Read the model definition and answer for the solid it produces. Units are mm, in the model's axes. Give positions to 0.01 mm unless a question says otherwise; leave off trailing zeros. Loops run counter-clockwise (first coordinate to the right, second up) from the corner with the lowest first, then second, coordinate; pieces in that order, holes last.
(1) Find section A-A, the plane z = 0. Write down the section's boundary in (x, y).
(2) Find section C-C, the plane z = 9.75. Write down the section's boundary in (x, y).
(3) Determine the mould class of faces 1 (the face through (2.88, -7.936, 0.018)), 2 (the face through (5.842, -3, 3)) for opening direction Z: pulls with the +Z half, pulls with the -Z half, needs draft (parallel to the pull), parting line crosses it, or undercut.
(4) Find section D-D, the plane z = -5.25. Write down the section's boundary in (x, y).
(5) Straight lines are drawn through the part: probe 1 along Y at (x, z) = (1.75, 0); probe 2 along Y at (x, z) = (5.2, 9.25); probe 3 along Z at (x, y) = (5.15, -6.25). For each, find the intervals that lie inside material, in ascending order.
(6) Find section B-B, the plane y = -10.5. Write down the section's boundary in (x, z), then the cut area to 3 significant figures.
```python
from build123d import *

# Parameters (mm, degrees)
BASPROSKE_W         = 5.842
BASPROSKE_H         = 12.7
TOOTHCUT_DEPTH      = 19.886740428
TEETHCUTS_COUNT     = 10
TEETHCUTS_ANGLE     = 324
BORSKE_R            = 3.175
BORE_DEPTH          = 50.8000508
SKETCH1_R           = 3.175
SKETCH1_R_2         = 2.921
BOSS_EXTRUDE1_DEPTH = 5.842


with BuildPart() as part:
    # BasProSke → Base-Revolve (revolve)
    with BuildSketch(Plane(origin=(0, 0, 0), x_dir=(1, 0, 0), z_dir=(0, 1, 0)), mode=Mode.PRIVATE) as base_revolve_sk:
        with Locations((2.921, 6.35)):
            Rectangle(BASPROSKE_W, BASPROSKE_H)
    revolve(base_revolve_sk.sketch.rotate(Axis((-10, 0, 0), (1, 0, 0)), 180), axis=Axis((-10, 0, 0), (1, 0, 0)))

    # TooCutSke → ToothCut (cut, through all)
    with BuildSketch(Plane(origin=(0, 0, 0), x_dir=(0, 0, -1), z_dir=(1, 0, 0))):
        with BuildLine():
            ThreePointArc((1.261053733, 7.835399804), (0, 7.93623), (-1.261053733, 7.835399804))
            ThreePointArc((-1.261053733, 7.835399804), (-1.789991322, 10.402889218), (-3.729263267, 12.166692264))
            ThreePointArc((-3.729263267, 12.166692264), (0, 12.7254), (3.729263267, 12.166692264))
            ThreePointArc((3.729263267, 12.166692264), (1.789991322, 10.402889218), (1.261053733, 7.835399804))
        make_face()
    toothcut = extrude(amount=TOOTHCUT_DEPTH, mode=Mode.SUBTRACT)

    # TeethCuts: ToothCut ×10 about axis
    teethcuts_axis = Axis((-10, 0, 0), (1, 0, 0))
    for i in range(1, TEETHCUTS_COUNT):
        add(toothcut.rotate(teethcuts_axis, i * TEETHCUTS_ANGLE / (TEETHCUTS_COUNT - 1)), mode=Mode.SUBTRACT)

    # BorSke → Bore (cut, symmetric)
    with BuildSketch(Plane(origin=(0, 0, 0), x_dir=(0, 0, -1), z_dir=(1, 0, 0))):
        with Locations(Location((0, 0, 0), (0, 0, 180))):
            Circle(BORSKE_R)
    extrude(amount=BORE_DEPTH, both=True, mode=Mode.SUBTRACT)

    # Sketch1 → Boss-Extrude1 (add)
    with BuildSketch(Plane(origin=(5.842, 0, 0), x_dir=(0, 0, -1), z_dir=(1, 0, 0))):
        Circle(SKETCH1_R)
        Circle(SKETCH1_R_2, mode=Mode.SUBTRACT)
    extrude(amount=-BOSS_EXTRUDE1_DEPTH)


solid = part.part
```
Entries:
1. outline: (0, -7.94) - (5.84, -7.94) - (5.84, -2.92) - (0, -2.92) - close; (0, 2.92) - (5.84, 2.92) - (5.84, 7.94) - (0, 7.94) - close
2. outline: (0, -7.72) - (5.84, -7.72) - (5.84, -5.44) - (0, -5.44) - close; (0, -1.6) - (5.84, -1.6) - (5.84, 1.6) - (0, 1.6) - close; (0, 5.44) - (5.84, 5.44) - (5.84, 7.72) - (0, 7.72) - close
3. face 1: undercut
3. face 2: needs draft
4. outline: (0, -5.95) - (5.84, -5.95) - (5.84, 5.95) - (0, 5.95) - close
5. probe 1: y = -7.94 to -2.92, 2.92 to 7.94
5. probe 2: y = -7.74 to -4.82, -1.59 to 1.59, 4.82 to 7.74
5. probe 3: z = -10.16 to -6.08, -4.89 to 4.89, 6.08 to 10.16
6. outline: (0, -4.65) - (5.84, -4.65) - (5.84, -1.85) - (0, -1.85) - close; (0, 1.85) - (5.84, 1.85) - (5.84, 4.65) - (0, 4.65) - close
6. area: 32.8 mm2
